from build123d import *

# Parameters (mm, degrees)
SKETCH_1_R          = 25
SKETCH_1_R_2        = 4
SKETCH_1_R_3        = 6
EXTRUDE_1_DEPTH     = 16
SKETCH_2_R          = 9
CUT_EXTRUDE_1_DEPTH = 12
SKETCH_3_R          = 2.5
CUT_EXTRUDE_2_DEPTH = 41
SKETCH_4_R          = 12.5
CUT_EXTRUDE_3_DEPTH = 12


with BuildPart() as part:
    # 草图1 → 凸台-拉伸1 (new body)
    with BuildSketch(Plane(origin=(0, 0, 0), x_dir=(1, 0, 0), z_dir=(0, 1, 0))):
        with BuildLine():
            Line((-125, 57.5), (125, 57.5))
            Line((125, 57.5), (125, -52.5))
            ThreePointArc((125, -52.5), (123.535533906, -56.035533906), (120, -57.5))
            Line((120, -57.5), (-120, -57.5))
            ThreePointArc((-120, -57.5), (-123.535533906, -56.035533906), (-125, -52.5))
            Line((-125, -52.5), (-125, 57.5))
        make_face()
        with Locations(Location((0, 0, 0), (0, 0, 270))):
            Circle(SKETCH_1_R, mode=Mode.SUBTRACT)
        with Locations(Location((69, -42, 0), (0, 0, 270))):
            Circle(SKETCH_1_R_2, mode=Mode.SUBTRACT)
        with Locations(Location((69, 42, 0), (0, 0, 90))):
            Circle(SKETCH_1_R_2, mode=Mode.SUBTRACT)
        with Locations(Location((-69, -42, 0), (0, 0, 90))):
            Circle(SKETCH_1_R_2, mode=Mode.SUBTRACT)
        with Locations(Location((-69, 42, 0), (0, 0, 270))):
            Circle(SKETCH_1_R_2, mode=Mode.SUBTRACT)
        with Locations(Location((30, 45, 0), (0, 0, 270))):
            Circle(SKETCH_1_R_3, mode=Mode.SUBTRACT)
        with Locations(Location((100, 45, 0), (0, 0, 270))):
            Circle(SKETCH_1_R_3, mode=Mode.SUBTRACT)
        with Locations(Location((-100, 45, 0), (0, 0, 90))):
            Circle(SKETCH_1_R_3, mode=Mode.SUBTRACT)
        with Locations(Location((-30, 45, 0), (0, 0, 90))):
            Circle(SKETCH_1_R_3, mode=Mode.SUBTRACT)
    extrude(amount=EXTRUDE_1_DEPTH)

    # 草图2 → 切除-拉伸1 (cut)
    with BuildSketch(Plane(origin=(0, 16, 0), x_dir=(1, 0, 0), z_dir=(0, 1, 0))):
        with Locations(Location((-100, 45, 0), (0, 0, 270))):
            Circle(SKETCH_2_R)
        with Locations(Location((-30, 45, 0), (0, 0, 270))):
            Circle(SKETCH_2_R)
        with Locations(Location((30, 45, 0), (0, 0, 90))):
            Circle(SKETCH_2_R)
        with Locations(Location((100, 45, 0), (0, 0, 90))):
            Circle(SKETCH_2_R)
    extrude(amount=-CUT_EXTRUDE_1_DEPTH, mode=Mode.SUBTRACT)

    # 草图3 → 切除-拉伸2 (cut)
    with BuildSketch(Plane(origin=(0, 16, 0), x_dir=(1, 0, 0), z_dir=(0, 1, 0))):
        with Locations(Location((-90, 0, 0), (0, 0, 270))):
            Circle(SKETCH_3_R)
        with Locations(Location((90, 0, 0), (0, 0, 270))):
            Circle(SKETCH_3_R)
    extrude(amount=-CUT_EXTRUDE_2_DEPTH, mode=Mode.SUBTRACT)

    # 草图4 → 切除-拉伸3 (cut)
    with BuildSketch(Plane.XZ):
        with Locations(Location((-90, 0, 0), (0, 0, 270))):
            Circle(SKETCH_4_R)
        with Locations(Location((90, 0, 0), (0, 0, 270))):
            Circle(SKETCH_4_R)
    extrude(amount=-CUT_EXTRUDE_3_DEPTH, mode=Mode.SUBTRACT)


solid = part.part
Model file for the job. Use its own axes, mm. A direction names the side the tool comes from. Coordinates: 2 decimals unless noted, no trailing zeros. Loops run counter-clockwise (first coordinate to the right, second up) from the corner with the lowest first, then second, coordinate; pieces in that order, holes last. Notation, with made-up numbers: (35, 1.5) -> (68, 1.5) arc R10 cw to (68, 20.5) -> close; hole circle Ø4 at (-30.5, 44.25). An arc over 180 degrees is marked (long way). Use one line per item in the form item = value. Start each with the question number.
(1) Cut at A-A on x = -69. Give the cut face in (y, z).
(2) Tool access for faces 4 (the flat face through (-93, 12, 0)), 5 (the cylindrical face through (108.786, 10.084, -43.049)), 6 (the flat face through (-125, 8, -2)): list every direction of +Z, -Z, +X, -X, +Y, -Y with a clear straight run to the whole face (end or side of a thin tool).
(3) Pull direction Z, two halves, no side cores. Call faces 1 (the cylindrical face through (123.57, 7.89, 56)), 2 (the flat face through (2, 0, -26)), 3 (the cylindrical face through (-72.905, 7.888, -42.867)): pulls with the +Z half, pulls with the -Z half, needs draft (parallel to the pull), parting line crosses it, or undercut.
(4) Flat gauge pins, fed straight in: pin 1 (9 mm diameter, centred on x = -69, z = 42, fed in from -Y); pin 2 (9 mm diameter, centred on x = 31, z = -41.5, fed in from +Y); pin 3 (7.5 mm diameter, centred on x = -90, z = 5, fed in from -Y). Where does each tip first touch, or does it go through?
(5) Cut at C-C on x = -100. Give the cut face in (y, z), and give its area (3 significant figures).
(6) Probe probe 1 along X at (y, z) = (13.7, 0); probe 2 along X at (y, z) = (14, 38.5); probe 3 along X at (y, z) = (9.5, -7.5). List the from-to ranges inside material, lowest first. Write a range as from..to.
(7) Cut at D-D on z = 0. Give the cut face in (x, y).
(8) Cut at B-B on z = 42. Give the cut face in (x, y).
Values:
q1.outline = (0, -57.5) -> (16, -57.5) -> (16, -46) -> (0, -46) -> close; (0, -38) -> (16, -38) -> (16, 38) -> (0, 38) -> close; (0, 46) -> (16, 46) -> (16, 57.5) -> (0, 57.5) -> close
q2.face_4 = -Y
q2.face_5 = +Y
q2.face_6 = +Z, -Z, -X, +Y, -Y
q3.face_1 = pulls with the +Z half
q3.face_2 = needs draft
q3.face_3 = undercut
q4.pin_1 = 0
q4.pin_2 = 4
q4.pin_3 = 12
q5.outline = (0, -57.5) -> (16, -57.5) -> (16, -54) -> (4, -54) -> (4, -51) -> (0, -51) -> close; (0, -39) -> (4, -39) -> (4, -36) -> (16, -36) -> (16, 57.5) -> (0, 57.5) -> (0, 7.5) -> (12, 7.5) -> (12, -7.5) -> (0, -7.5) -> close
q5.area = 1,400 mm2
q6.probe_1 = -125..-92.5, -87.5..-25, 25..87.5, 92.5..125
q6.probe_2 = -125..-70.94, -67.06..67.06, 70.94..125
q6.probe_3 = -125..-100, -80..-23.85, 23.85..80, 100..125
q7.outline = (-125, 0) -> (-102.5, 0) -> (-102.5, 12) -> (-92.5, 12) -> (-92.5, 16) -> (-125, 16) -> close; (-87.5, 12) -> (-77.5, 12) -> (-77.5, 0) -> (-25, 0) -> (-25, 16) -> (-87.5, 16) -> close; (25, 0) -> (77.5, 0) -> (77.5, 12) -> (87.5, 12) -> (87.5, 16) -> (25, 16) -> close; (92.5, 12) -> (102.5, 12) -> (102.5, 0) -> (125, 0) -> (125, 16) -> (92.5, 16) -> close
q8.outline = (-125, 0) -> (-73, 0) -> (-73, 16) -> (-125, 16) -> close; (-65, 0) -> (65, 0) -> (65, 16) -> (-65, 16) -> close; (73, 0) -> (125, 0) -> (125, 16) -> (73, 16) -> close
